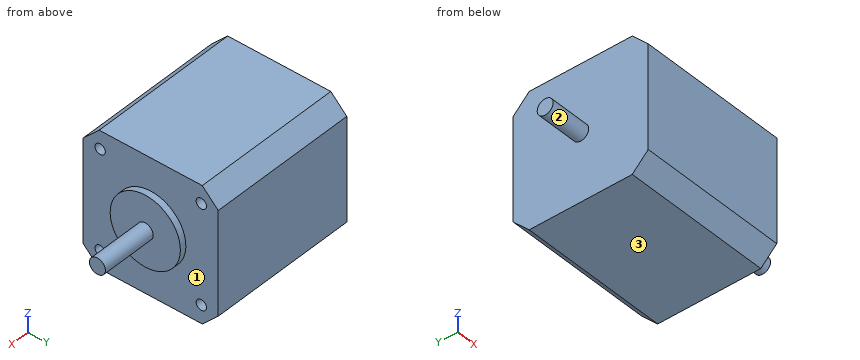
Autodesk Inventor part; units mm, degrees
ref_plane "YZ Plane" through (0, 0, 0) normal (1, 0, 0) x (0, 1, 0)
ref_plane "XZ Plane" through (0, 0, 0) normal (0, 1, 0) x (-1, 0, 0)
ref_plane "XY Plane" through (0, 0, 0) normal (0, 0, 1) x (1, 0, 0)
sketch "Sketch1" plane through (0, 0, 0) normal (1, 0, 0) x (0, 1, 0)
  line L0 (0, 0) -> (42.3, 0)
  line L1 (42.3, 0) -> (42.3, 42.3)
  line L2 (42.3, 42.3) -> (0, 42.3)
  line L3 (0, 42.3) -> (0, 0)
  dimension "d0" = 42.3
  dimension "d1" = 42.3
extrude "Extrusion1" add sketch "Sketch1" along normal blind 47
sketch "Sketch2" plane through (47, 0, 0) normal (1, 0, 0) x (0, 0, -1)
  circle A0 centre (-21.15, 21.15) radius 11
  dimension "d4" = 22
extrude "Extrusion2" add sketch "Sketch2" along normal blind 2
sketch "Sketch3" plane through (47, 0, 0) normal (1, 0, 0) x (0, 0, -1)
  line L0 (-36.65, 5.3) -> (-5.65, 37) construction
  line L1 (-5.65, 5.3) -> (-36.65, 37) construction
  point P0 (-21.15, 21.15)
  point P1 (-21.15, 21.15)
  point P2 (-21.15, 21.15)
  dimension "d7" = 31
hole "Hole1" at (47, 21.15, 21.15) at (47, 37, 36.65) at (47, 37, 5.65) at (47, 5.3, 5.65) at (47, 5.3, 36.65) direction (-1, 0, 0) diameter 3.242 depth 4.5
chamfer "Chamfer1" distance 5 angle 45 4 edges at (23.5, 42.3, 42.3) (23.5, 42.3, 0) (23.5, 0, 42.3) (23.5, 0, 0)
sketch "Sketch4" plane through (49, 21.15, 21.15) normal (1, 0, 0) x (0, 0, -1)
  circle A0 centre (0, 0) radius 11
  circle A1 centre (0, 0) radius 2.5
  point P0 (21.15, -21.15)
  dimension "d18" = 5
extrude "Extrusion3" add sketch "Sketch4" along normal blind 17.5 contours A1
sketch "Sketch5" plane through (0, 0, 0) normal (-1, 0, 0) x (0, 0, 1)
  circle A0 centre (21.15, 21.15) radius 2.5
  point P0 (0, 0)
  dimension "d21" = 5
extrude "Extrusion4" add sketch "Sketch5" along normal blind 13
properties part number "NEMA17-dual-shaft"
Work out the finished part from the listing and answer in its coordinate system (mm). Face numbers are marked on the shaded views. A direction names the side the tool comes from. Give positions to 0.01 mm unless a question says otherwise; leave off trailing zeros. Loops run counter-clockwise (first coordinate to the right, second up) from the corner with the lowest first, then second, coordinate; pieces in that order, holes last. Notation, with made-up numbers: (65.5, -14) -> (71.5, -14) arc R23 ccw to (71.5, 21) -> close; hole circle Ø11 at (45, -31.5). An arc over 180 degrees is marked (long way). Use CSV: the item, a comma, the result in double quotes.
1. Straight lines are drawn through the part: line 1 (Y direction, x = 45.95, z = 5.65); line 2 (Z direction, x = 44.4, y = 5.3); line 3 (Z direction, x = 45.3, y = 21.15). For each, find the intervals that lie inside material, in ascending order.
Found:
line 1,"0 to 3.68, 6.92 to 35.38, 38.62 to 42.3"
line 2,"0 to 4.03, 7.27 to 35.03, 38.27 to 42.3"
line 3,"0 to 19.53, 22.77 to 42.3"
2. Flat-ended cylindrical pins translate along their axes: pin 1 Ø3.5 at (y, z) = (36.5, 37.5) entering from +X; pin 2 Ø1 at (y, z) = (11, 36) entering from -X; pin 3 Ø2.5 at (y, z) = (5.3, 5.65) entering from +X. Find the tip coordinate at first contact, or state that the pin passes through.
Found:
pin 1,"x = 47"
pin 2,"x = 0"
pin 3,"x = 42.5"
3. The part is cut by section C-C (x = 11). Write down the section's boundary in (y, z).
Found:
outline,"(0, 5) -> (5, 0) -> (37.3, 0) -> (42.3, 5) -> (42.3, 37.3) -> (37.3, 42.3) -> (5, 42.3) -> (0, 37.3) -> close"
4. The part is cut by section D-D (z = 26). Write down the section's boundary in (x, y), then the cut area to 3 significant figures.
Found:
outline,"(0, 0) -> (47, 0) -> (47, 11.28) -> (49, 11.28) -> (49, 31.02) -> (47, 31.02) -> (47, 42.3) -> (0, 42.3) -> close"
area,"2,030 mm^2"
5. The part is cut by section A-A (z = 21.15). Write down the section's boundary in (x, y), then the cut area to 3 significant figures.
Found:
outline,"(-13, 18.65) -> (0, 18.65) -> (0, 0) -> (47, 0) -> (47, 10.15) -> (49, 10.15) -> (49, 18.65) -> (66.5, 18.65) -> (66.5, 23.65) -> (49, 23.65) -> (49, 32.15) -> (47, 32.15) -> (47, 42.3) -> (0, 42.3) -> (0, 23.65) -> (-13, 23.65) -> close; hole (42.5, 19.53) -> (47, 19.53) -> (47, 22.77) -> (42.5, 22.77) -> close"
area,"2,170 mm^2"
6. A tool of negligible diameter and unlimited length cuts with its end or side. For the marked faces 1, 2 and 3, from which of +Z, -Z, +X, -X, +Y, -Y can it reach the whole face along a straight path? Write none if from no direction.
Found:
face 1,"+X"
face 2,"-X"
face 3,"-Z, +X, -X, +Y, -Y"
